```python
from build123d import *

# Parameters (mm, degrees)
F0_R         = 135
F1_DEPTH     = 330.2
F1_TAPER     = -3
F2_R         = 134.8030624247
F3_DEPTH     = 292.1
F3_TAPER     = 3
F4_R         = 156.9952990324
F5_DEPTH     = 25
F6_R         = 146.995306015
F6_W         = 52
F6_H         = 52
F6_R_2       = 3.1
F7_DEPTH     = 20
F7_FACE_R    = 146.995306015
F7_FACE1_R   = 156.9952990324
F7_FACE1_R_2 = 146.995306015
F8_DEPTH     = 10
F8_TAPER     = 86
F9_DEPTH     = 254


with BuildPart() as f1:
    # F0 (on Top) → F1 (new body)
    with BuildSketch(Plane.XY):
        Circle(F0_R)
    extrude(amount=F1_DEPTH, taper=F1_TAPER)

    # F2 (on face) → F3 (cut)
    with BuildSketch(Plane.XY.offset(330.2)):
        Circle(F2_R)
    extrude(amount=-F3_DEPTH, taper=F3_TAPER, mode=Mode.SUBTRACT)

    # F4 (on face) → F5 (join)
    with BuildSketch(Plane.XY.offset(330.2)):
        Circle(F4_R)
    extrude(amount=F5_DEPTH)

    # F6 (on face) → F7 (cut)
    with BuildSketch(Plane.XY.offset(355.2)):
        Circle(F6_R)
        with Locations((-69.1615422964, 5.5897118747)):
            Rectangle(F6_W, F6_H, mode=Mode.SUBTRACT)
        Circle(F6_R_2, mode=Mode.SUBTRACT)
        with Locations((83.9149872065, 2.1923439801)):
            Rectangle(F6_W, F6_H, mode=Mode.SUBTRACT)
        with Locations((83.9149872065, 2.1923439801)):
            Rectangle(F6_W, F6_H)
        with Locations((-69.1615422964, 5.5897118747)):
            Rectangle(F6_W, F6_H)
        Circle(F6_R_2)
    extrude(amount=-F7_DEPTH, mode=Mode.SUBTRACT)

    # F7_face (on face) + F7_face1 (on face) → F8 (join)
    with BuildSketch(Plane.XY.offset(335.2)):
        Circle(F7_FACE_R)
    with BuildSketch(Plane.XY.offset(355.2)):
        Circle(F7_FACE1_R)
        Circle(F7_FACE1_R_2, mode=Mode.SUBTRACT)
    extrude(amount=F8_DEPTH, taper=F8_TAPER)

    # F6 (on face) → F9 (cut)
    with BuildSketch(Plane.XY.offset(355.2)):
        with Locations((83.9149872065, 2.1923439801)):
            Rectangle(F6_W, F6_H)
        with Locations((-69.1615422964, 5.5897118747)):
            Rectangle(F6_W, F6_H)
        Circle(F6_R_2)
    extrude(amount=-F9_DEPTH, mode=Mode.SUBTRACT)


solid = f1.part
```
Read the model definition and answer for the solid it produces. Units are mm, in the model's axes. A direction names the side the tool comes from. Give positions to 0.01 mm unless a question says otherwise; leave off trailing zeros. Order: outer loops, then holes, each group sorted by start corner. A loop starts at its lowest first (then second) coordinate and runs counter-clockwise, first axis right, second up.
(1) Straight lines are drawn through the part: L1, parallel to Y at x = 0, z = 335; L2, parallel to Y at x = 0, z = 349.75; L3, parallel to Z at x = 73, y = 31. For each, find the intervals that lie inside material, in ascending order.
(2) For a pull along Y with two mould halves and no side action, classify faces 5 (the flat face through (-2, 2, 0)), 6 (the flat face through (-2, 2, 38.1)), 7 (the flat face through (-70, 31.59, 335)) as released by +Y, released by -Y, zero draft, split by the parting line, or undercut.
(3) For faces 1 (the flat face through (-43.162, 5, 336)), 2 (the flat face through (-2, -28, 330.2)), 3 (the flat face through (-129, 82, 330.2)), 4 (the cylindrical face through (-34.034, -153.262, 342.525)), determine the directions among +Z, -Z, +X, -X, +Y, -Y from which every point of the face is accessible in a straight line to the end or side of a thin tool.
(4) Find section A-A (z = 273). Give the vertices of the cut face in (x, y), plus the area to 3 significant figures.
(5) Find section B-B (z = 170). Give the vertices of the cut face in (x, y).
(6) Given pin 1 (10 mm diameter, centred on x = -3, y = -72.5, fed in from +Z); pin 2 (2 mm diameter, centred on y = -81, z = 277.5, fed in from -X); pin 3 (9 mm diameter, centred on x = -68.5, z = 333, fed in from -Y), each flat-ended and moving along its own axis, determine where each tip first touches the part or whether it passes through.
Result sheet:
1. L1: y = -157 to -3.1, 3.1 to 157
1. L2: y = -157 to -147, 147 to 157
1. L3: z = 0 to 38.1, 330.2 to 339.93
2. face 5: zero draft
2. face 6: undercut
2. face 7: undercut
3. face 1: +Z
3. face 2: none
3. face 3: -Z
3. face 4: +Z, -Z
4. outline: circle Ø298.61 at (0, 0); hole circle Ø263.61 at (0, 0)
4. area: 15,500 mm2
5. outline: circle Ø287.82 at (0, 0); hole circle Ø252.81 at (0, 0)
6. pin 1: stops at z = 340.75
6. pin 2: stops at x = -126.35
6. pin 3: stops at y = -143.36
